Source: CAD feature listing. Evaluate the final solid. Frame: model axes, mm. Round coordinates to 2 decimals unless told otherwise and drop trailing zeros. Loops run counter-clockwise (first coordinate to the right, second up) from the corner with the lowest first, then second, coordinate; pieces in that order, holes last. Notation, with made-up numbers: M 17.25,39 L 22.25,39 A20 ccw 22.25,71 Z; hole C -36.5,-20 d1. An arc over 180 degrees is marked long. Answer as a JSON object with one key per item and string values.
from build123d import *

# Parameters (mm, degrees)
F0_W     = 768.35
F0_H     = 25.4
F1_DEPTH = 25.4
F2_W     = 22.225
F2_H     = 22.225
F3_DEPTH = 768.351
F5_DEPTH = 565.15


with BuildPart() as f1:
    # F0 (on Top) → F1 (new body)
    with BuildSketch(Plane.XY):
        Rectangle(F0_W, F0_H)
    extrude(amount=F1_DEPTH)

    # F2 (on face) → F3 (cut, through all)
    with BuildSketch(Plane.YZ.offset(384.175)):
        with Locations((1.5875, 11.1125)):
            Rectangle(F2_W, F2_H)
    extrude(amount=-F3_DEPTH, mode=Mode.SUBTRACT)

    # F4 (on face) → F5 (join)
    with BuildSketch(Plane.XY.offset(25.4)):
        Polygon((384.175, -12.7), (384.175, 12.7), (381, 12.7), (381, -9.525), (358.775, -9.525), (358.775, -12.7), align=None)
    extrude(amount=-F5_DEPTH)

    # F6: F1 across plane


with BuildPart() as f1_1:
    add(f1.part)
    add(f1.part.mirror(Plane.YZ))


solid = f1_1.part
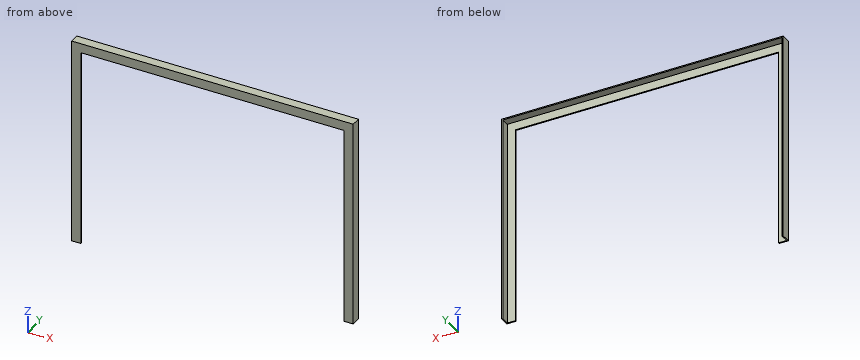
Item 1: Section B-B on y = 0.5. Return the cut outline in (x, z) (3 decimals).
Answer sheet:
{"outline": "M -384.175,-539.75 L -381,-539.75 L -381,22.225 L 381,22.225 L 381,-539.75 L 384.175,-539.75 L 384.175,25.4 L -384.175,25.4 Z"}
Item 2: Line query: probe 1 along X at (y, z) = (-11.5, -51.5) (3 decimals); probe 2 along X at (y, z) = (-4.5, -225.5) (3 decimals); probe 3 along Z at (x, y) = (-330, -6.75) (3 decimals). Output: solid intervals per line, ascending. Write a range as from..to.
Answer sheet:
{"probe 1": "x = -384.175..-358.775, 358.775..384.175", "probe 2": "x = -384.175..-381, 381..384.175", "probe 3": "z = 22.225..25.4"}
Item 3: Section A-A on z = -91. Return the cut outline in (x, y) (3 decimals), then the cut area to 3 significant figures.
Answer sheet:
{"outline": "M -384.175,-12.7 L -358.775,-12.7 L -358.775,-9.525 L -381,-9.525 L -381,12.7 L -384.175,12.7 Z; M 358.775,-12.7 L 384.175,-12.7 L 384.175,12.7 L 381,12.7 L 381,-9.525 L 358.775,-9.525 Z", "area": "302 mm²"}
Item 4: Section C-C on x = 254. Return the cut outline in (y, z) (3 decimals).
Answer sheet:
{"outline": "M -12.7,0 L -9.525,0 L -9.525,22.225 L 12.7,22.225 L 12.7,25.4 L -12.7,25.4 Z"}
Item 5: Contact query for a flat-ended pin moving along its axis: pin 1 Ø1 at (x, y) = (-44, -11) entering from -Z. Output: stop coordinate, or through.
Answer sheet:
{"pin 1": "stops at z = 0"}
